The model under review builds one solid part; all positions refer to its coordinate system, in mm. Coordinates: 2 decimals unless noted, no trailing zeros. Order: outer loops, then holes, each group sorted by start corner. A loop starts at its lowest first (then second) coordinate and runs counter-clockwise, first axis right, second up. Notation, with made-up numbers: (19, 57) - (76, 57) arc R22 cw to (76, 76) - close; hole circle Ø10 at (64, 44). An arc over 180 degrees is marked (long way). Answer in a Markdown table with one row per item.
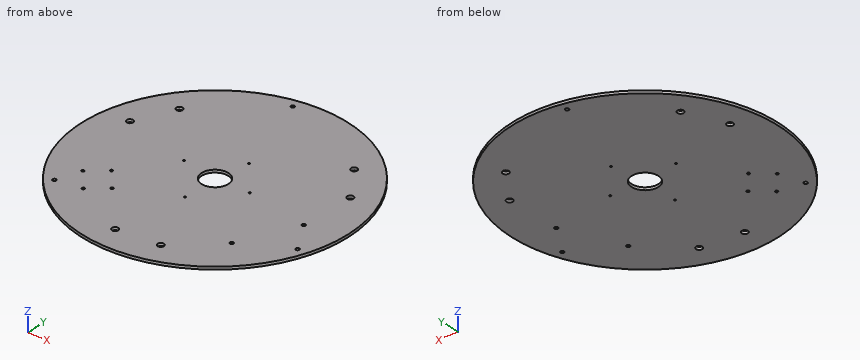
```python
from build123d import *

# Parameters (mm, degrees)
SKETCH1_R           = 150
BOSS_EXTRUDE1_DEPTH = 3
SKETCH2_R           = 3.5
CUT_EXTRUDE1_DEPTH  = 3
CIRPATTERN1_COUNT   = 3
SKETCH3_R           = 2
CUT_EXTRUDE2_DEPTH  = 3
SKETCH4_R           = 15
CUT_EXTRUDE3_DEPTH  = 3
SKETCH5_R           = 1
CUT_EXTRUDE4_DEPTH  = 3
SKETCH6_R           = 1.5
CUT_EXTRUDE5_DEPTH  = 3
SKETCH7_R           = 2
CUT_EXTRUDE6_DEPTH  = 3
CIRPATTERN2_COUNT   = 3


with BuildPart() as part:
    # Sketch1 → Boss-Extrude1 (new body)
    with BuildSketch(Plane.XY):
        Circle(SKETCH1_R)
    extrude(amount=BOSS_EXTRUDE1_DEPTH)

    # Sketch2 → Cut-Extrude1 (cut)
    with BuildSketch(Plane(origin=(0, 0, 0), x_dir=(-1, 0, 0), z_dir=(0, 0, -1))):
        with Locations((-84.532410842, 88.488821425)):
            Circle(SKETCH2_R)
        with Locations(Location((-112.064079787, 49.169523299, 0), (0, 0, 180))):
            Circle(SKETCH2_R)
    cut_extrude1 = extrude(amount=-CUT_EXTRUDE1_DEPTH, mode=Mode.SUBTRACT)

    # CirPattern1: Cut-Extrude1 ×3 about axis
    cirpattern1_axis = Axis((0, 0, 0), (0, 0, 1))
    for i in range(1, CIRPATTERN1_COUNT):
        add(cut_extrude1.rotate(cirpattern1_axis, i * 360 / CIRPATTERN1_COUNT), mode=Mode.SUBTRACT)

    # Sketch3 → Cut-Extrude2 (cut)
    with BuildSketch(Plane(origin=(0, 0, 0), x_dir=(-1, 0, 0), z_dir=(0, 0, -1))):
        with Locations((-109.9539568, -12.654144936)):
            Circle(SKETCH3_R)
        with Locations((-80.370678478, -76.095690029)):
            Circle(SKETCH3_R)
    extrude(amount=-CUT_EXTRUDE2_DEPTH, mode=Mode.SUBTRACT)

    # Sketch4 → Cut-Extrude3 (cut)
    with BuildSketch(Plane(origin=(0, 0, 0), x_dir=(-1, 0, 0), z_dir=(0, 0, -1))):
        Circle(SKETCH4_R)
    extrude(amount=-CUT_EXTRUDE3_DEPTH, mode=Mode.SUBTRACT)

    # Sketch5 → Cut-Extrude4 (cut)
    with BuildSketch(Plane(origin=(0, 0, 0), x_dir=(-1, 0, 0), z_dir=(0, 0, -1))):
        with Locations((0.451473383, -40.846457118)):
            Circle(SKETCH5_R)
        with Locations((-38.922466014, 0.285726101)):
            Circle(SKETCH5_R)
        with Locations((40.304305183, 6.648298355)):
            Circle(SKETCH5_R)
        with Locations((-7.040200573, 38.28153048)):
            Circle(SKETCH5_R)
    extrude(amount=-CUT_EXTRUDE4_DEPTH, mode=Mode.SUBTRACT)

    # Sketch6 → Cut-Extrude5 (cut)
    with BuildSketch(Plane(origin=(0, 0, 0), x_dir=(-1, 0, 0), z_dir=(0, 0, -1))):
        with Locations((59.302185735, -69.341551519)):
            Circle(SKETCH6_R)
        with Locations((78.453296813, -85.411241761)):
            Circle(SKETCH6_R)
        with Locations((97.736925104, -62.429908467)):
            Circle(SKETCH6_R)
        with Locations((78.585814026, -46.360218225)):
            Circle(SKETCH6_R)
    extrude(amount=-CUT_EXTRUDE5_DEPTH, mode=Mode.SUBTRACT)

    # Sketch7 → Cut-Extrude6 (cut)
    with BuildSketch(Plane(origin=(0, 0, 0), x_dir=(-1, 0, 0), z_dir=(0, 0, -1))):
        with Locations((107.246222037, -89.990265356)):
            Circle(SKETCH7_R)
    cut_extrude6 = extrude(amount=-CUT_EXTRUDE6_DEPTH, mode=Mode.SUBTRACT)

    # CirPattern2: Cut-Extrude6 ×3 about axis
    cirpattern2_axis = Axis((0, 0, 0), (0, 0, 1))
    for i in range(1, CIRPATTERN2_COUNT):
        add(cut_extrude6.rotate(cirpattern2_axis, i * 360 / CIRPATTERN2_COUNT), mode=Mode.SUBTRACT)


solid = part.part
```
Item 1: We need section C-C, the plane y = 59.5. Write out the cut boundary in (x, z), then the cut area to 3 significant figures.
Check values:
| item | result |
|---|---|
| outline | (-137.69, 0) - (137.69, 0) - (137.69, 3) - (-137.69, 3) - close |
| area | 826 mm^2 |
Item 2: We need section B-B, the plane y = -131. Write out the cut boundary in (x, z).
Check values:
| item | result |
|---|---|
| outline | (-73.07, 0) - (73.07, 0) - (73.07, 3) - (-73.07, 3) - close |
Item 3: To check wall thickness, follow line 1 (Y direction, x = 33, z = 2.4); line 2 (X direction, y = 12, z = 1); line 3 (X direction, y = 10, z = 0.7). State the ranges of each line that lie inside material, in increasing order. Write a range as from..to.
Check values:
| item | result |
|---|---|
| line 1 | -146.32..-120.67, -114.23..146.32 |
| line 2 | -149.52..-9, 9..149.52 |
| line 3 | -149.67..-11.18, 11.18..149.67 |
Item 4: We need section A-A, the plane z = 1.55. State how many separate pieces and enclosed holes the cut face has, then the cut area to 3 significant figures.
Check values:
| item | result |
|---|---|
| separate pieces | 1 |
| enclosed holes | 20 |
| area | 69,600 mm^2 |
